Verification items for the finished model (mm, model axes). A direction names the side the tool comes from. Coordinates: 2 decimals unless noted, no trailing zeros. Order: outer loops, then holes, each group sorted by start corner. A loop starts at its lowest first (then second) coordinate and runs counter-clockwise, first axis right, second up. Notation, with made-up numbers: M 52,87 L 71,87 A19 ccw 71,114 Z; hole C 84.25,44.5 d7. An arc over 180 degrees is marked long. Return JSON: item names as keys, results as strings.
```python
from build123d import *

# Parameters (mm, degrees)
BOSS_EXTRUDE1_DEPTH      = 10
BOSS_EXTRUDE1_DEPTH_BACK = 10
CUT_EXTRUDE1_DEPTH       = 8
CUT_EXTRUDE2_DEPTH       = 57.402570863
CUT_EXTRUDE2_DEPTH_BACK  = 57.402570863
SKETCH4_R                = 1.75


with BuildPart() as part:
    # Sketch1 → Boss-Extrude1 (new, two sides: drawn at the far end of the back side and taken through both)
    with BuildSketch(Plane.XY.offset(-BOSS_EXTRUDE1_DEPTH_BACK)):
        with BuildLine():
            Line((7.5, -15), (7.5, 15))
            Line((7.5, 15), (7.5, 55))
            Line((7.5, 55), (5.024246851, 55))
            ThreePointArc((5.024246851, 55), (3.811940358, 54.590695749), (3.095836066, 53.530312966))
            Line((3.095836066, 53.530312966), (-7.5, 15))
            Line((-7.5, 15), (-7.5, -15))
            Line((-7.5, -15), (7.5, -15))
        make_face()
        Polygon((7, 15.5), (-6.843938287, 15.5), (-4.918938287, 22.5), (7, 22.5), align=None, mode=Mode.SUBTRACT)
        Polygon((7, 30), (7, 23), (-4.781438287, 23), (-2.856438287, 30), align=None, mode=Mode.SUBTRACT)
        Polygon((7, 37.5), (7, 30.5), (-2.718938287, 30.5), (-0.793938287, 37.5), align=None, mode=Mode.SUBTRACT)
        Polygon((7, 38), (-0.656438287, 38), (1.268561713, 45), (7, 45), align=None, mode=Mode.SUBTRACT)
        with BuildLine():
            ThreePointArc((3.476897778, 53.030312966), (4.193002071, 54.090695749), (5.405308564, 54.5))
            Line((5.405308564, 54.5), (7, 54.5))
            Line((7, 54.5), (7, 45.5))
            Line((7, 45.5), (1.406061713, 45.5))
            Line((1.406061713, 45.5), (3.476897778, 53.030312966))
        make_face(mode=Mode.SUBTRACT)
    extrude(amount=BOSS_EXTRUDE1_DEPTH + BOSS_EXTRUDE1_DEPTH_BACK)

    # Sketch2 → Cut-Extrude1 (cut)
    with BuildSketch(Plane.XY.offset(10)):
        Polygon((5.5, 7.378745231), (5.5, 15.378745231), (0.5, 15.378745231), (-4.5, 10.378745231), (-4.5, -15.621254769), (4.5, -15.621254769), (0.5, -11.621254769), (0.5, 2.378745231), align=None)
    cut_extrude1 = extrude(amount=-CUT_EXTRUDE1_DEPTH, mode=Mode.SUBTRACT)

    # Mirror1: Cut-Extrude1 across plane
    add(cut_extrude1.mirror(Plane.XY), mode=Mode.SUBTRACT)

    # Sketch4 → Cut-Extrude2 (cut, two sides: drawn at the far end of the back side and taken through both)
    with BuildSketch(Plane.XY.offset(-CUT_EXTRUDE2_DEPTH_BACK)):
        with Locations((1.5, 9.378745231)):
            Circle(SKETCH4_R)
    extrude(amount=CUT_EXTRUDE2_DEPTH + CUT_EXTRUDE2_DEPTH_BACK, mode=Mode.SUBTRACT)


solid = part.part
```
Q1. Cross-section at C-C, the plane y = 6.5. Record the boundary of the cut face in (x, z).
Values:
{"outline": "M -7.5,-10 L -4.5,-10 L -4.5,-2 L 4.62,-2 L 4.62,-10 L 7.5,-10 L 7.5,10 L 4.62,10 L 4.62,2 L -4.5,2 L -4.5,10 L -7.5,10 Z"}
Q2. Tool access check on faces 1 (the face through (5.5, 11, -6)), 2 (the face through (3.826, 54.602, -0.14)), 3 (the face through (6, 54.5, 0)). Record the directions out of +Z, -Z, +X, -X, +Y, -Y that give a thin tool (end or side, any length) a straight path to the whole face; none if there is none.
Values:
{"face 1": "-Z", "face 2": "+Z, -Z, -X, +Y", "face 3": "+Z, -Z"}
Q3. Material ranges on line 1 along X through (y, z) = (-5.5, -3); line 2 along X through (y, z) = (7.5, 9.25); line 3 along Z through (x, y) = (-1, -5.5), recorded low to high.
Values:
{"line 1": "-7.5 to -4.5, 0.5 to 7.5", "line 2": "-7.5 to -4.5, 5.5 to 7.5", "line 3": "-2 to 2"}
Q4. Cross-section at B-B, the plane z = 3. State how many separate pieces and enclosed holes the cut face has, and give its area (3 significant figures).
Values:
{"separate pieces": "1", "enclosed holes": "5", "area": "319 mm^2"}
Q5. Cross-section at A-A, the plane y = 50.5. Record the boundary of the cut face in (x, z), and give its area (3 significant figures).
Values:
{"outline": "M 2.26,-10 L 2.78,-10 L 2.78,10 L 2.26,10 Z; M 7,-10 L 7.5,-10 L 7.5,10 L 7,10 Z", "area": "20.4 mm^2"}
Q6. Go/stop test with flat-tipped pins: pin 1 (2 mm diameter, centred on y = 32.5, z = 1.5, fed in from -X); pin 2 (1.5 mm diameter, centred on x = -3, z = -6, fed in from -Y); pin 3 (5.5 mm diameter, centred on y = 18, z = 2, fed in from -X); pin 4 (4 mm diameter, centred on x = 4, z = -7, fed in from +Y). Record where each tip stops, or that it passes through.
Values:
{"pin 1": "x = -2.96", "pin 2": "y = 11.13", "pin 3": "x = -7.43", "pin 4": "y = 55"}
Q7. Draft check along Y on faces 4 (the face through (7.5, 20, 0)), 5 (the face through (2.21, -13.33, 6.06)), 6 (the face through (1.272, 11.114, -0.028)). Enter one of: pulls with the +Y half, pulls with the -Y half, needs draft (parallel to the pull), parting line crosses it, or undercut.
Values:
{"face 4": "needs draft", "face 5": "pulls with the -Y half", "face 6": "undercut"}
